Verification items for this drawing (mm, ordinates from the low corner). Give positions to 0.01 mm unless a question says otherwise; leave off trailing zeros. Loops run counter-clockwise (first coordinate to the right, second up) from the corner with the lowest first, then second, coordinate; pieces in that order, holes last. Notation, with made-up numbers: M 72,-39.75 L 83,-39.75 A21 cw 83,-27.75 Z; hole C 49,69.25 d4. An arc over 180 degrees is marked long. Use a Markdown table: item, result.
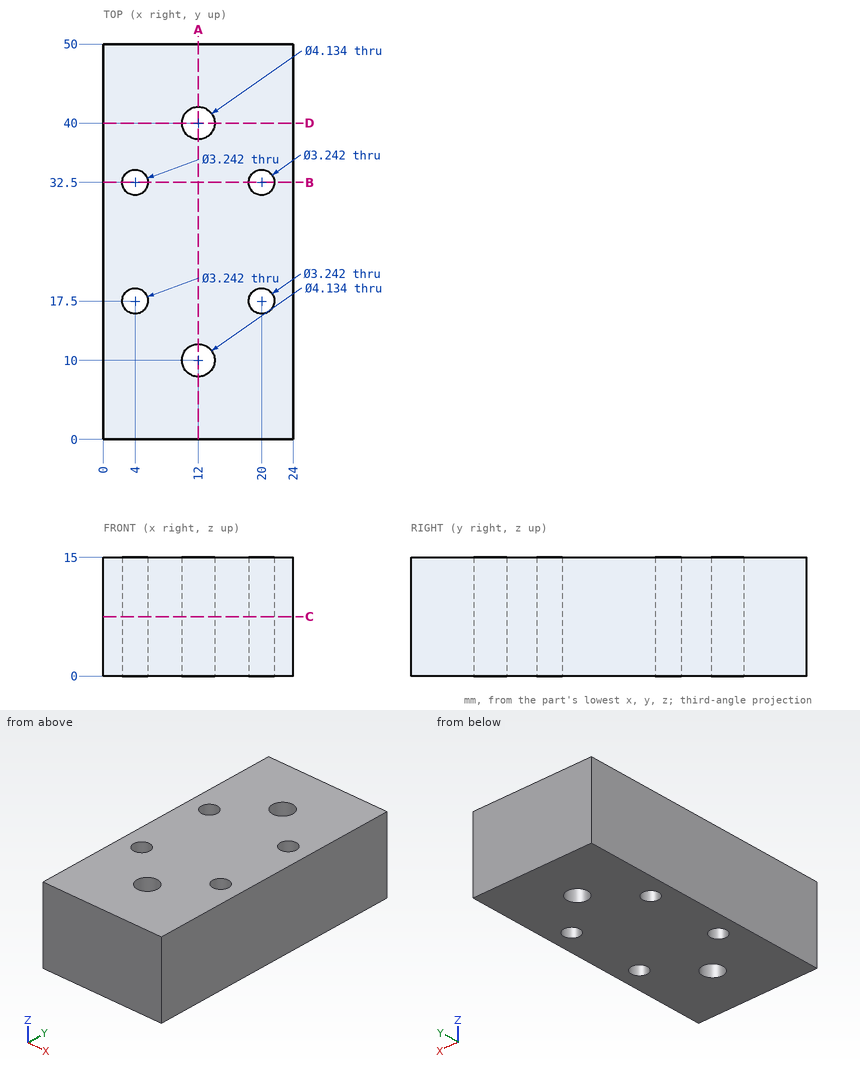
(1) Cross-section at D-D on y = 40. Record the cut outline in (x, z).
Results below:
| item | result |
|---|---|
| outline | M 0,0 L 9.93,0 L 9.93,15 L 0,15 Z; M 14.07,0 L 24,0 L 24,15 L 14.07,15 Z |
(2) Material ranges on line 1 (Y direction, x = 12, z = 5.75); line 2 (X direction, y = 32.5, z = 12.25); line 3 (Y direction, x = 4, z = 3.5), recorded low to high.
Results below:
| item | result |
|---|---|
| line 1 | 0 to 7.93, 12.07 to 37.93, 42.07 to 50 |
| line 2 | 0 to 2.38, 5.62 to 18.38, 21.62 to 24 |
| line 3 | 0 to 15.88, 19.12 to 30.88, 34.12 to 50 |
(3) Gauge pin test, flat end, axial feed: P1, Ø2.5, axis at x = 12, y = 10, coming from the +Z side. Record the tip position at first contact, or that the pin passes through.
Results below:
| item | result |
|---|---|
| P1 | through |
(4) Cross-section at A-A on x = 12. Record the cut outline in (y, z), then the cut area to 3 significant figures.
Results below:
| item | result |
|---|---|
| outline | M 0,0 L 7.93,0 L 7.93,15 L 0,15 Z; M 12.07,0 L 37.93,0 L 37.93,15 L 12.07,15 Z; M 42.07,0 L 50,0 L 50,15 L 42.07,15 Z |
| area | 626 mm^2 |
(5) Cross-section at B-B on y = 32.5. Record the cut outline in (x, z), then the cut area to 3 significant figures.
Results below:
| item | result |
|---|---|
| outline | M 0,0 L 2.38,0 L 2.38,15 L 0,15 Z; M 5.62,0 L 18.38,0 L 18.38,15 L 5.62,15 Z; M 21.62,0 L 24,0 L 24,15 L 21.62,15 Z |
| area | 263 mm^2 |
(6) Cross-section at C-C on z = 7.5. Record the cut outline in (x, y), then the cut area to 3 significant figures.
Results below:
| item | result |
|---|---|
| outline | M 0,0 L 24,0 L 24,50 L 0,50 Z; hole C 4,17.5 d3.24; hole C 4,32.5 d3.24; hole C 12,10 d4.13; hole C 12,40 d4.13; hole C 20,17.5 d3.24; hole C 20,32.5 d3.24 |
| area | 1,140 mm^2 |
